The listing builds one solid part. Answer for the finished solid, in the listing's coordinates (mm). Face numbers are marked on the shaded views. A direction names the side the tool comes from. Round coordinates to 2 decimals unless told otherwise and drop trailing zeros. Order: outer loops, then holes, each group sorted by start corner. A loop starts at its lowest first (then second) coordinate and runs counter-clockwise, first axis right, second up. Notation, with made-up numbers: (14.5, 78) -> (41.5, 78) arc R34 ccw to (41.5, 112) -> close; hole circle Ø3 at (-10, 9). An arc over 180 degrees is marked (long way). Return JSON: item names as keys, results as strings. Group by question number.
(1) Which of the six approach directions +Z, -Z, +X, -X, +Y, -Y give full straight-line access (tool end or side, diameter ignored) to the marked faces 1 and 2?
(2) The part is cut by section C-C (x = -2.2). Determine the outline of the cut face in (y, z).
(3) The part is cut by section A-A (z = -2.5). Determine the outline of the cut face in (x, y).
(4) Consider line 1 (X direction, y = -0.05, z = -3.75); line 2 (X direction, y = -0.65, z = -2); line 3 (Y direction, x = -0.9, z = 1.25). Determine where each line is inside the solid, lowest interval first. Write a range as [from, to].
(5) Each of these flat-tipped pins is pushed along its axis until it touches: pin 1 (0.8 mm diameter, centred on y = 0, z = 1, fed in from -X) (3 decimals); pin 2 (1.5 mm diameter, centred on y = 0, z = -4.5, fed in from -X); pin 3 (3 mm diameter, centred on x = -1.5, z = -3, fed in from -Y). Where does it stop, or does it pass through?
(6) The part is cut by section B-B (x = 1.55). Determine the outline of the cut face in (y, z), plus the area to 3 significant figures.
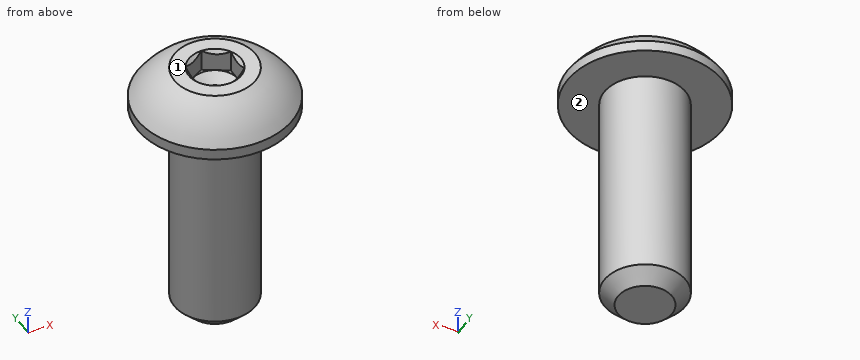
from build123d import *

# Parameters (mm, degrees)
SKETCH1_W          = 7.9375
SKETCH1_H          = 1.4224
CHAMFER1_SIZE      = 0.47625
SKETCH4_R          = 2.7051
EXTRUDE1_DEPTH     = 1.4986
CUT_EXTRUDE1_DEPTH = 0.7493
SKETCH7_R          = 0.916543552
CUT_EXTRUDE4_DEPTH = 0.7493
CUT_EXTRUDE4_TAPER = 45
SKETCH8_R          = 0.79375
CUT_EXTRUDE5_DEPTH = 0.249766667
CUT_EXTRUDE5_TAPER = 60


with BuildPart() as part:
    # Sketch1 → Revolve1 (revolve)
    with BuildSketch(Plane(origin=(0, 0, 0), x_dir=(0, 0, -1), z_dir=(1, 0, 0))):
        with Locations((3.96875, 0.7112)):
            Rectangle(SKETCH1_W, SKETCH1_H)
    revolve(axis=Axis((0, 0, 0), (0, 0, 1)))

    # Chamfer1
    chamfer1_edges = [part.edges().sort_by_distance(p)[0] for p in [
        (0, -1.4224, -7.9375),
    ]]
    chamfer(chamfer1_edges, length=CHAMFER1_SIZE)

    # Sketch4 → Extrude1 (add)
    with BuildSketch(Plane.XY):
        Circle(SKETCH4_R)
    extrude(amount=EXTRUDE1_DEPTH)

    # Sketch9 → Cut-Revolve3 (revolve, cut)
    with BuildSketch(Plane(origin=(0, 0, 0), x_dir=(0, 0, -1), z_dir=(1, 0, 0))):
        with BuildLine():
            Line((0, 2.7051), (-0.381, 2.7051))
            ThreePointArc((-0.381, 2.7051), (-1.025093234, 2.138064897), (-1.4986, 1.4224))
            Line((-1.4986, 1.4224), (-1.8796, 1.4224))
            Line((-1.8796, 1.4224), (-1.8796, 3.0861))
            Line((-1.8796, 3.0861), (0, 3.0861))
            Line((0, 3.0861), (0, 2.7051))
        make_face()
    revolve(axis=Axis((0, 0, 0), (0, 0, 1)), mode=Mode.SUBTRACT)

    # Sketch6 → Cut-Extrude1 (cut)
    with BuildSketch(Plane.XY.offset(1.4986)):
        Polygon((0, -0.916543552), (0.79375, -0.458271776), (0.79375, 0.458271776), (0, 0.916543552), (-0.79375, 0.458271776), (-0.79375, -0.458271776), align=None)
    extrude(amount=-CUT_EXTRUDE1_DEPTH, mode=Mode.SUBTRACT)

    # Sketch7 → Cut-Extrude4 (cut)
    with BuildSketch(Plane.XY.offset(1.4986)):
        Circle(SKETCH7_R)
    extrude(amount=-CUT_EXTRUDE4_DEPTH, taper=CUT_EXTRUDE4_TAPER, mode=Mode.SUBTRACT)

    # Sketch8 → Cut-Extrude5 (cut)
    with BuildSketch(Plane.XY.offset(0.7493)):
        Circle(SKETCH8_R)
    extrude(amount=-CUT_EXTRUDE5_DEPTH, taper=CUT_EXTRUDE5_TAPER, mode=Mode.SUBTRACT)


solid = part.part
Answer below:
{
 "1": {"face 1": "+Z, +X, -X, +Y, -Y", "face 2": "-Z"},
 "2": {"outline": "(-1.57, 0) -> (1.57, 0) -> (1.57, 0.38) arc R2.4 ccw to (-1.57, 0.38) -> close"},
 "3": {"outline": "circle Ø2.84 at (0, 0)"},
 "4": {"line 1": "x = [-1.42, 1.42]", "line 2": "x = [-1.27, 1.27]", "line 3": "y = [-1.61, 1.61]"},
 "5": {"pin 1": "stops at x = -2.545", "pin 2": "stops at x = -1.42", "pin 3": "stops at y = -1.42"},
 "6": {"outline": "(-2.22, 0) -> (2.22, 0) -> (2.22, 0.38) arc R2.86 ccw to (-2.22, 0.38) -> close", "area": "4.94 mm²"}
}
